```python
from build123d import *

# Parameters (mm, degrees)
F0_R     = 2.399673
F1_DEPTH = 2.54
F3_DEPTH = 25.4
F5_DEPTH = 25.4


with BuildPart() as f1:
    # F0 (on Front) → F1 (new body)
    with BuildSketch(Plane.XZ):
        with BuildLine():
            Line((50.793077, 7.724595), (-9.531923, 7.724595))
            Line((-9.531923, 7.724595), (-9.531923, -11.325405))
            Line((-9.531923, -11.325405), (-0.006923, -11.325405))
            Line((-0.006923, -11.325405), (-0.000719, -4.049985))
            Line((-0.000719, -4.049985), (-0.001371, -7.724225))
            ThreePointArc((-0.001371, -7.724225), (2.248548, -2.188908), (7.721398, 0.208962))
            Line((7.721398, 0.208962), (50.793077, 1.374595))
            Line((50.793077, 1.374595), (50.793077, 7.724595))
        make_face()
        with Locations((-4.112308, 2.531883)):
            Circle(F0_R, mode=Mode.SUBTRACT)
    extrude(amount=F1_DEPTH)

    # F2 (on face) → F3 (cut)
    with BuildSketch(Plane(origin=(-9.531923, 0, 0), x_dir=(0, -1, 0), z_dir=(-1, 0, 0))):
        Polygon((2.54, -11.325405), (2.54, 0), (0.716685, -11.325405), align=None)
    extrude(amount=-F3_DEPTH, mode=Mode.SUBTRACT)

    # F4 (on face) → F5 (cut)
    with BuildSketch(Plane.XY.offset(7.724595)):
        Polygon((50.793077, 0), (36.557514, 0), (50.793077, -1.016), align=None)
        Polygon((50.793077, -1.524), (36.557514, -2.54), (50.793077, -2.54), align=None)
    extrude(amount=-F5_DEPTH, mode=Mode.SUBTRACT)


solid = f1.part
```
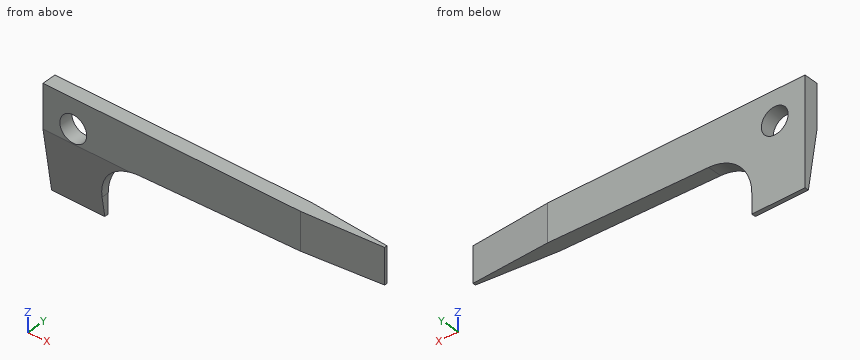
CAD build for the part. Positions are in the model's coordinates, mm. Round coordinates to 2 decimals unless told otherwise and drop trailing zeros. Loops run counter-clockwise (first coordinate to the right, second up) from the corner with the lowest first, then second, coordinate; pieces in that order, holes last. Notation, with made-up numbers: M 70,76 L 103,76 A8 ccw 103,90 Z; hole C -11,20 d10. An arc over 180 degrees is marked long. Return JSON: item names as keys, results as strings. Group by question number.
(1) Wall check: probe 1 along Y at (x, z) = (-1.5, -6.25); probe 2 along Z at (x, y) = (17.5, -1.75); probe 3 along Z at (x, y) = (32, -1.8). Give the ranges that are in metal, low to high. Write a range as [from, to].
(2) Drop flat-ended pins along their axis: P1, Ø1.5, axis at y = -1, z = -8, coming from the +X side; P2, Ø1.5, axis at y = -1, z = -5, coming from the +X side. Give the stop position or say it passes through.
(3) Saw through at C-C, the plane x = 2. List the corners of the cut face in (y, z), and give its area (3 significant figures).
(4) Saw through at A-A, the plane z = 3.5. List the corners of the cut face in (x, y).
(5) Saw through at B-B, the plane z = 5.75. List the corners of the cut face in (x, y), and give its area (3 significant figures).
Answer list:
{
 "1": {"probe 1": "[-1.53, 0]", "probe 2": "[0.47, 7.72]", "probe 3": "[0.87, 7.72]"},
 "2": {"P1": "x = 0.01", "P2": "x = 0.8"},
 "3": {"outline": "M -2.54,0 L -2.14,-2.46 L 0,-2.46 L 0,7.72 L -2.54,7.72 Z", "area": "25.4 mm2"},
 "4": {"outline": "M -9.53,-2.54 L -6.31,-2.54 L -6.31,0 L -9.53,0 Z; M -1.92,-2.54 L 36.56,-2.54 L 50.79,-1.52 L 50.79,-1.02 L 36.56,0 L -1.92,0 Z"},
 "5": {"outline": "M -9.53,-2.54 L 36.56,-2.54 L 50.79,-1.52 L 50.79,-1.02 L 36.56,0 L -9.53,0 Z", "area": "139 mm2"}
}
